Model file for the job. Use its own axes, mm. A direction names the side the tool comes from. Round coordinates to 2 decimals unless told otherwise and drop trailing zeros. Write each loop counter-clockwise with the first axis right and the second up, starting at its lowest first coordinate (ties: lowest second). Pieces come first, ordered by that corner, then holes. Notation, with made-up numbers: (50.5, 45.5) - (74.5, 45.5) arc R25 ccw to (74.5, 58.5) - close; hole circle Ø11 at (21.5, 79.25). An arc over 180 degrees is marked (long way). One line per item, written item: value.
from build123d import *

# Parameters (mm, degrees)
SKETCH1_R               = 11
BOSS_EXTRUDE1_DEPTH     = 10
SKETCH1_3_R             = 7.5
BOSS_EXTRUDE2_DEPTH     = 7
SKETCH1_4_R             = 2.5
CUT_EXTRUDE1_DEPTH      = 10
CUT_EXTRUDE1_DEPTH_BACK = 11


with BuildPart() as part:
    # Sketch1 → Boss-Extrude1 (new body)
    with BuildSketch(Plane(origin=(0, 0, 0), x_dir=(1, 0, 0), z_dir=(0, 1, 0))):
        Circle(SKETCH1_R)
    extrude(amount=-BOSS_EXTRUDE1_DEPTH)

    # Sketch1_3 → Boss-Extrude2 (add)
    with BuildSketch(Plane(origin=(0, 0, 0), x_dir=(1, 0, 0), z_dir=(0, 1, 0))):
        Circle(SKETCH1_3_R)
    extrude(amount=BOSS_EXTRUDE2_DEPTH)

    # Sketch1_4 → Cut-Extrude1 (cut, two sides)
    with BuildSketch(Plane(origin=(0, 0, 0), x_dir=(1, 0, 0), z_dir=(0, 1, 0))) as cut_extrude1_sk:
        Circle(SKETCH1_4_R)
    extrude(amount=CUT_EXTRUDE1_DEPTH, mode=Mode.SUBTRACT)
    extrude(cut_extrude1_sk.sketch, amount=-CUT_EXTRUDE1_DEPTH_BACK, mode=Mode.SUBTRACT)


solid = part.part
1. Band-saw the part on A-A on x = 0. Write the cut outline in (y, z).
Report:
outline: (-10, -11) - (0, -11) - (0, -7.5) - (7, -7.5) - (7, -2.5) - (-10, -2.5) - close; (-10, 2.5) - (7, 2.5) - (7, 7.5) - (0, 7.5) - (0, 11) - (-10, 11) - close
2. Wall check: probe 1 along X at (y, z) = (-3.5, 0); probe 2 along Z at (x, y) = (0, 3.75). Give the ranges that are in metal, low to high. Write a range as [from, to].
Report:
probe 1: [-11, -2.5], [2.5, 11]
probe 2: [-7.5, -2.5], [2.5, 7.5]
3. Band-saw the part on C-C on y = -8.5. Write the cut outline in (x, z).
Report:
outline: circle Ø22 at (0, 0); hole circle Ø5 at (0, 0)
4. Drop flat-ended pins along their axis: pin 1 (12 mm diameter, centred on x = 7, z = 4, fed in from +Y); pin 2 (1 mm diameter, centred on y = -6.5, z = -1.5, fed in from +X); pin 3 (5 mm diameter, centred on x = 4.5, y = -0.5, fed in from -Z); pin 4 (2 mm diameter, centred on y = -3.5, z = 4, fed in from +X). Give the stop position or say it passes through.
Report:
pin 1: y = 7
pin 2: x = 10.95
pin 3: z = -10.82
pin 4: x = 10.58
5. Band-saw the part on B-B on z = 0. Write the cut outline in (x, y), plus the area to 3 significant figures.
Report:
outline: (-11, -10) - (-2.5, -10) - (-2.5, 7) - (-7.5, 7) - (-7.5, 0) - (-11, 0) - close; (2.5, -10) - (11, -10) - (11, 0) - (7.5, 0) - (7.5, 7) - (2.5, 7) - close
area: 240 mm²
6. Tool access for faces 4 (the face through (7.2, 0, -2.6)), 5 (the face through (-2, 7, -2)): list every direction of +Z, -Z, +X, -X, +Y, -Y with a clear straight run to the whole face (end or side of a thin tool).
Report:
face 4: +Y
face 5: +Z, -Z, +X, -X, +Y
7. Band-saw the part on D-D on x = -6.75. Write the cut outline in (y, z), plus the area to 3 significant figures.
Report:
outline: (-10, -8.69) - (0, -8.69) - (0, -3.27) - (7, -3.27) - (7, 3.27) - (0, 3.27) - (0, 8.69) - (-10, 8.69) - close
area: 219 mm²
8. Mould opens along Z. For faces 1 (the face through (-2.38, -4.93, 10.74)), 2 (the face through (-0.54, -1.38, 2.44)), 3 (the face through (-3, -10, 0)) say: released by +Z, released by -Z, zero draft, split by the parting line, or undercut.
Report:
face 1: split by the parting line
face 2: undercut
face 3: zero draft
